Source: three-view drawing plus pictorial views. Frame: mm from the lowest corner of the part. A direction names the side the tool comes from. Give positions to 0.01 mm unless a question says otherwise; leave off trailing zeros. Write each loop counter-clockwise with the first axis right and the second up, starting at its lowest first coordinate (ties: lowest second). Pieces come first, ordered by that corner, then holes.
Q1. Pin query (flat end, axial travel): pin 1 (15 mm diameter, centred on x = 38.5, y = 35.5, fed in from +Z); pin 2 (22 mm diameter, centred on x = 37.5, y = 24, fed in from -Z); pin 3 (2.5 mm diameter, centred on x = 2.5, z = 15, fed in from -Y); pin 4 (4.5 mm diameter, centred on y = 38.56, z = 30, fed in from -X). Return the tip coordinate at first contact, or that it passes through.
Q2. Cut plane D-D on y = 97.5. Return the cut outline in (x, z), plus the area to 3 significant figures.
Q3. Cut plane B-B on z = 54. Return the cut outline in (x, y).
Q4. Line query: L1, parallel to Y at x = 50, z = 30 (3 decimals); L2, parallel to Y at x = 50.5, z = 30 (3 decimals); L3, parallel to Z at x = 24.5, y = 32.5. Output: solid intervals per line, ascending.
Q5. Reachability of the marked faces 4, 5 and 6 from +Z, -Z, +X, -X, +Y, -Y: full face, straight path, thin tool, end or side. Return the list, or none.
Q6. Draft query along Y for the marked faces 1, 2 and 3. Return one class per face: pulls with the +Y half, pulls with the -Y half, needs draft (parallel to the pull), parting line crosses it, or undercut.
Q7. Cut plane C-C on x = 30. Return the cut outline in (y, z).
Q8. Cut plane A-A on y = 21.56. Return the cut outline in (x, z).
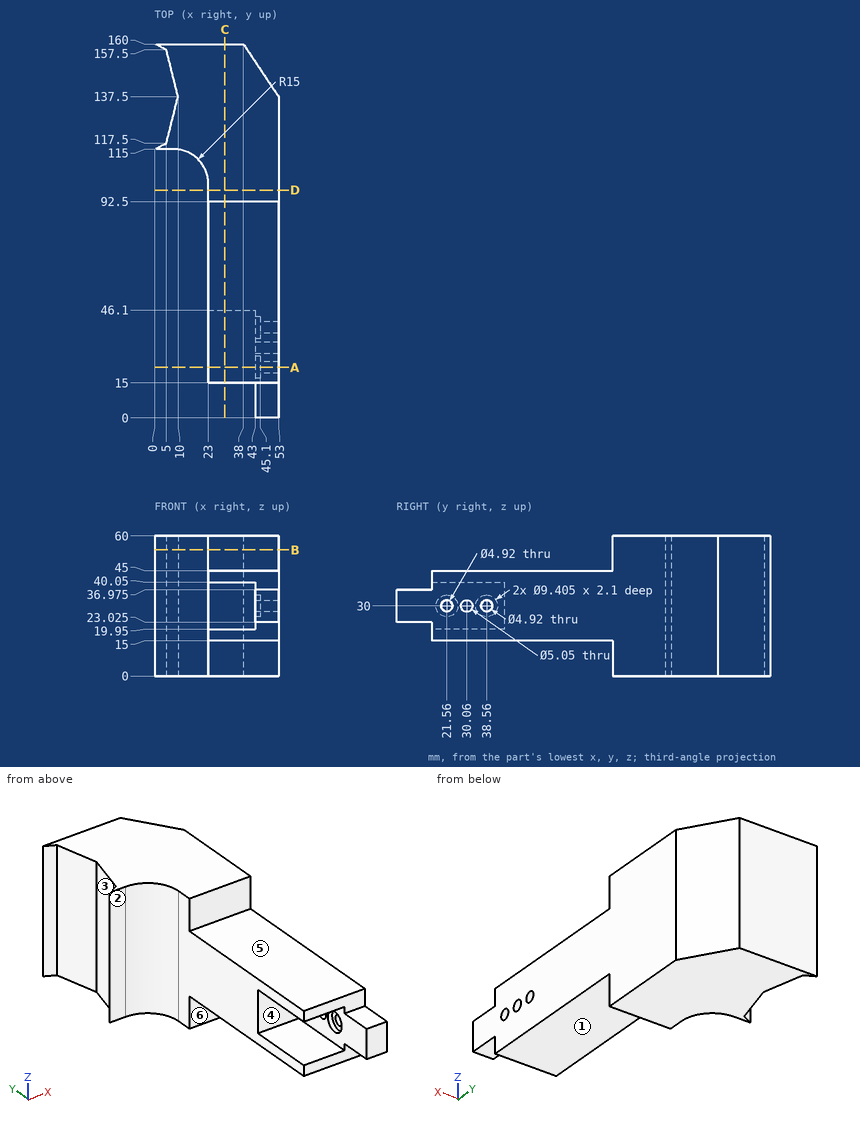
Data:
1. pin 1: stops at z = 45
1. pin 2: stops at z = 15
1. pin 3: stops at y = 115
1. pin 4: passes through
2. outline: (23, 0) - (53, 0) - (53, 60) - (23, 60) - close
2. area: 1,800 mm2
3. outline: (0, 115) - (8, 115) arc R15 cw to (23, 100) - (23, 92.5) - (53, 92.5) - (53, 137.5) - (38, 160) - (0, 160) - (5, 157.5) - (10, 137.5) - (5, 117.5) - close
4. L1: y = 0 to 19.1, 24.02 to 27.535, 32.585 to 36.1, 41.02 to 142
4. L2: y = 0 to 19.1, 24.02 to 27.535, 32.585 to 36.1, 41.02 to 141.25
4. L3: z = 15 to 19.95, 40.05 to 45
5. face 4: -X, -Y
5. face 5: +Z, +X, -X, -Y
5. face 6: -Z, +X, -X, -Y
6. face 1: needs draft
6. face 2: pulls with the -Y half
6. face 3: undercut
7. outline: (15, 15) - (92.5, 15) - (92.5, 0) - (160, 0) - (160, 60) - (92.5, 60) - (92.5, 45) - (15, 45) - (15, 40.05) - (46.1, 40.05) - (46.1, 19.95) - (15, 19.95) - close
8. outline: (23, 15) - (53, 15) - (53, 27.54) - (45.1, 27.54) - (45.1, 25.3) - (43, 25.3) - (43, 19.95) - (23, 19.95) - close; (23, 40.05) - (43, 40.05) - (43, 34.7) - (45.1, 34.7) - (45.1, 32.46) - (53, 32.46) - (53, 45) - (23, 45) - close
